Autodesk Inventor part; units mm, degrees
ref_plane "XZ Plane" through (0, 0, 0) normal (0, 1, 0) x (-1, 0, 0)
ref_plane "XY Plane" through (0, 0, 0) normal (0, 0, 1) x (1, 0, 0)
sketch "Sketch1" plane through (0, 0, 0) normal (0, 1, 0) x (-1, 0, 0)
  line L0 (-35, 52.5) -> (35, 52.5)
  line L1 (35, 52.5) -> (35, -52.5)
  line L2 (35, -52.5) -> (-35, -52.5)
  line L3 (-35, -52.5) -> (-35, 52.5)
  line L4 (-35, 52.5) -> (35, -52.5) construction
  line L5 (35, 52.5) -> (-35, -52.5) construction
  point P0 (0, 0)
  dimension "d0" = 105
  dimension "d1" = 70
extrude "Extrusion1" add sketch "Sketch1" along normal blind 40
fillet "Fillet1" radius 10 4 edges at (-35, 20, 52.5) (35, 20, 52.5) (-35, 20, -52.5) (35, 20, -52.5)
sketch "Sketch2" plane through (0, 40, 0) normal (0, 1, 0) x (1, 0, 0)
  line L0 (29, -37.5) -> (-29, -37.5)
  line L1 (-29, -37.5) -> (-29, 37.5)
  line L2 (-29, 37.5) -> (29, 37.5)
  line L3 (29, 37.5) -> (29, -37.5)
  line L4 (29, -37.5) -> (-29, 37.5) construction
  line L5 (-29, -37.5) -> (29, 37.5) construction
  point P0 (0, 0)
  dimension "d5" = 58
  dimension "d6" = 75
extrude "Extrusion2" cut sketch "Sketch2" against normal blind 38
properties part number "CH_01_0038_kradex_place_holder"
Could you check a few things on this model? Use its own coordinates, in mm. A direction names the side the tool comes from. Give positions to 0.01 mm unless a question says otherwise; leave off trailing zeros. Write each loop counter-clockwise with the first axis right and the second up, starting at its lowest first coordinate (ties: lowest second). Pieces come first, ordered by that corner, then holes. Notation, with made-up numbers: (-1, 4) -> (20, 4) arc R20 ccw to (20, 8) -> close; hole circle Ø10 at (74, 52). An arc over 180 degrees is marked (long way). Answer as a JSON object with one key per item and string values.
Q1. Suppose I cut it at D-D on z = -46. Write out the boundary of the cut face in (x, y), then the cut area to 3 significant figures.
Taken from the geometry:
{"outline": "(-34.37, 0) -> (34.37, 0) -> (34.37, 40) -> (-34.37, 40) -> close", "area": "2,750 mm²"}
Q2. Suppose I cut it at A-A on z = -13.5. Write out the boundary of the cut face in (x, y), then the cut area to 3 significant figures.
Taken from the geometry:
{"outline": "(-35, 0) -> (35, 0) -> (35, 40) -> (29, 40) -> (29, 2) -> (-29, 2) -> (-29, 40) -> (-35, 40) -> close", "area": "596 mm²"}
Q3. We'd pull the mould along X, two halves only. Please class faces 3 (the flat face through (35, 20, -1)), 4 (the flat face through (0, 2, -1)), 5 (the flat face through (-35, 20, 1)): released by +X, released by -X, zero draft, split by the parting line, or undercut.
Taken from the geometry:
{"face 3": "released by +X", "face 4": "undercut", "face 5": "released by -X"}
Q4. Suppose I cut it at C-C on x = -1. Write out the boundary of the cut face in (y, z), then the cut area to 3 significant figures.
Taken from the geometry:
{"outline": "(0, -52.5) -> (40, -52.5) -> (40, -37.5) -> (2, -37.5) -> (2, 37.5) -> (40, 37.5) -> (40, 52.5) -> (0, 52.5) -> close", "area": "1,350 mm²"}
Q5. Which directions (+Z, -Z, +X, -X, +Y, -Y) give clear straight access to the entire face, cutting with the end or side of a thin tool? Please do faces 1 (the cylindrical face through (32.15, 20.28, -49.49)), 2 (the flat face through (29, 21, -1)).
Taken from the geometry:
{"face 1": "-Z, +X, +Y, -Y", "face 2": "+Y"}
Q6. Suppose I cut it at B-B on y = 36. Write out the boundary of the cut face in (x, z), then the cut area to 3 significant figures.
Taken from the geometry:
{"outline": "(-35, -42.5) arc R10 ccw to (-25, -52.5) -> (25, -52.5) arc R10 ccw to (35, -42.5) -> (35, 42.5) arc R10 ccw to (25, 52.5) -> (-25, 52.5) arc R10 ccw to (-35, 42.5) -> close; hole (-29, -37.5) -> (29, -37.5) -> (29, 37.5) -> (-29, 37.5) -> close", "area": "2,910 mm²"}
Q7. Please list where these lines run through material, in increasing order: L1, parallel to Z at x = -23.5, y = 21; L2, parallel to X at y = 18, z = -23.5; L3, parallel to Y at x = -10, z = -8.5.
Taken from the geometry:
{"L1": "z = -52.5 to -37.5, 37.5 to 52.5", "L2": "x = -35 to -29, 29 to 35", "L3": "y = 0 to 2"}
Q8. Will this pin go through, and if not, where does the flat tip stop? pin 1 Ø1 at (x, z) = (-3.5, 16.5) entering from +Y.
Taken from the geometry:
{"pin 1": "stops at y = 2"}
